from build123d import *

# Parameters (mm, degrees)
EXTRUDE_1_DEPTH                = 4
CUT_EXTRUDE_1_DEPTH            = 105.27847333
CUT_EXTRUDE_1_DEPTH_BACK       = 105.27847333
SKETCH_2_R                     = 2
SKETCH_2_W                     = 4
SKETCH_2_H                     = 16
CHAMFER_1_SIZE                 = 1
CUT_EXTRUDE_2_DEPTH            = 105.27847333
CUT_EXTRUDE_2_DEPTH_BACK       = 105.27847333
SKETCH_6_W                     = 20
SKETCH_6_H                     = 5
EXTRUDE_2_DEPTH                = 25
CHAMFER_2_SIZE                 = 1
EXTRUDE_START                  = -5
EXTRUDE_3_DEPTH                = 5
SKETCH_8_R                     = 6
EXTRUDE_4_DEPTH                = 5
CHAMFER_3_SIZE                 = 1
SKETCH_9_R                     = 4
EXTRUDE_5_DEPTH                = 5
CUT_EXTRUDE_START              = -10
SKETCH_10_R                    = 2
CUT_EXTRUDE_3_DEPTH            = 120.608393839
HOLE_WIZARD_1_4_0_15748031_1_D = 3.999999874
SKETCH_13_R                    = 1.5
CUT_EXTRUDE_4_DEPTH            = 109.434311913
SKETCH_14_R                    = 2
CUT_EXTRUDE_5_DEPTH            = 109.434311913
CUT_EXTRUDE_START_2            = 10
SKETCH_15_R                    = 4
CUT_EXTRUDE_6_DEPTH            = 10
CHAMFER_4_SIZE                 = 2
CHAMFER_5_SIZE                 = 1
SKETCH_16_W                    = 18
SKETCH_16_H                    = 4
CUT_EXTRUDE_7_DEPTH            = 109.434311913
SKETCH_17_R                    = 1.5
EXTRUDE_6_DEPTH                = 3


with BuildPart() as part:
    # 草图1 → 凸台-拉伸1 (new body)
    with BuildSketch(Plane(origin=(0, 0, 0), x_dir=(1, 0, 0), z_dir=(0, 1, 0))):
        Polygon((0, -34), (0, 34), (17, 47), (32, 47), (32, 34), (55, 34), (55, 47), (61, 47), (63, 45), (93, 45), (93, -45), (63, -45), (61, -47), (55, -47), (55, -34), (32, -34), (32, -47), (17, -47), align=None)
    extrude(amount=EXTRUDE_1_DEPTH)

    # 草图2 → 切除-拉伸1 (cut, two sides: drawn at the far end of the back side and taken through both)
    with BuildSketch(Plane(origin=(0, 4, 0), x_dir=(1, 0, 0), z_dir=(0, 1, 0)).offset(-CUT_EXTRUDE_1_DEPTH_BACK)):
        with Locations(Location((13, 10, 0), (0, 0, 270))):
            Circle(SKETCH_2_R)
        with Locations(Location((13, -10, 0), (0, 0, 90))):
            Circle(SKETCH_2_R)
        with Locations((6, 0)):
            Rectangle(SKETCH_2_W, SKETCH_2_H)
        Polygon((4, 12), (4, 26), (17, 36.408329997), (17, 33.205766921), (8, 26), (8, 12), align=None)
        Polygon((8, -26), (8, -12), (4, -12), (4, -26), (17, -36.408329997), (17, -33.205766921), align=None)
    extrude(amount=CUT_EXTRUDE_1_DEPTH + CUT_EXTRUDE_1_DEPTH_BACK, mode=Mode.SUBTRACT)

    # 倒角1
    chamfer_1_edges = [part.edges().sort_by_distance(p)[0] for p in [
        (8.5, 4, 40.5),
        (24.5, 4, 47),
        (8.5, 4, -40.5),
        (24.5, 4, -47),
        (0, 4, 0),
    ]]
    chamfer(chamfer_1_edges, length=CHAMFER_1_SIZE)

    # 草图3 → 切除-拉伸2 (cut, two sides: drawn at the far end of the back side and taken through both)
    with BuildSketch(Plane(origin=(0, 4, 0), x_dir=(1, 0, 0), z_dir=(0, 1, 0)).offset(-CUT_EXTRUDE_2_DEPTH_BACK)):
        Polygon((93, 22), (33, 22), (21, 10), (21, -10), (33, -22), (93, -22), align=None)
    extrude(amount=CUT_EXTRUDE_2_DEPTH + CUT_EXTRUDE_2_DEPTH_BACK, mode=Mode.SUBTRACT)

    # 草图6 → 凸台-拉伸2 (add)
    with BuildSketch(Plane(origin=(0, 4, 0), x_dir=(1, 0, 0), z_dir=(0, 1, 0))):
        with BuildLine():
            Line((21, 10), (21, 15))
            ThreePointArc((21, 15), (15, 21), (21, 27))
            Line((21, 27), (33, 27))
            Line((33, 27), (33, 22))
            Line((33, 22), (21, 10))
        make_face()
        with Locations((83, 24.5)):
            Rectangle(SKETCH_6_W, SKETCH_6_H)
    extrude_2 = extrude(amount=EXTRUDE_2_DEPTH)

    # 镜向1: 凸台-拉伸2 across plane
    add(extrude_2.mirror(Plane.XY))

    # 倒角2
    chamfer_2_edges = [part.edges().sort_by_distance(p)[0] for p in [
        (83, 4, -27),
        (73, 4, -24.5),
        (83, 4, 27),
        (73, 4, 24.5),
    ]]
    chamfer(chamfer_2_edges, length=CHAMFER_2_SIZE)

    # 草图7 → 凸台-拉伸3 (add)
    with BuildSketch(Plane(origin=(0, 29, 0), x_dir=(1, 0, 0), z_dir=(0, 1, 0)).offset(EXTRUDE_START)):
        with BuildLine():
            Line((93, 22), (93, 27))
            Line((93, 27), (73, 27))
            Line((73, 27), (73, 21))
            Line((73, 21), (53, 21))
            Line((53, 21), (53, 27))
            Line((53, 27), (33, 27))
            Line((33, 27), (21, 27))
            ThreePointArc((21, 27), (15, 21), (21, 15))
            Line((21, 15), (21, 10))
            Line((21, 10), (21, -10))
            Line((21, -10), (21, -15))
            ThreePointArc((21, -15), (15, -21), (21, -27))
            Line((21, -27), (33, -27))
            Line((33, -27), (53, -27))
            Line((53, -27), (53, -21))
            Line((53, -21), (73, -21))
            Line((73, -21), (73, -27))
            Line((73, -27), (93, -27))
            Line((93, -27), (93, -22))
            Line((93, -22), (93, 22))
        make_face()
    extrude(amount=EXTRUDE_3_DEPTH)

    # 草图8 → 凸台-拉伸4 (add)
    with BuildSketch(Plane(origin=(0, 29, 0), x_dir=(1, 0, 0), z_dir=(0, 1, 0))):
        with Locations(Location((21, 21, 0), (0, 0, 270))):
            Circle(SKETCH_8_R)
        with Locations(Location((21, -21, 0), (0, 0, 270))):
            Circle(SKETCH_8_R)
    extrude(amount=EXTRUDE_4_DEPTH)

    # 倒角3
    chamfer_3_edges = [part.edges().sort_by_distance(p)[0] for p in [
        (21, 34, -27),
        (21, 34, 15),
    ]]
    chamfer(chamfer_3_edges, length=CHAMFER_3_SIZE)

    # 草图9 → 凸台-拉伸5 (add)
    with BuildSketch(Plane(origin=(0, 29, 0), x_dir=(1, 0, 0), z_dir=(0, 1, 0))):
        with Locations(Location((83, 21, 0), (0, 0, 270))):
            Circle(SKETCH_9_R)
    extrude_5 = extrude(amount=EXTRUDE_5_DEPTH)

    # 草图10 → 切除-拉伸3 (cut)
    with BuildSketch(Plane(origin=(0, 34, 0), x_dir=(1, 0, 0), z_dir=(0, 1, 0)).offset(CUT_EXTRUDE_START)):
        with Locations(Location((83, 21, 0), (0, 0, 270))):
            Circle(SKETCH_10_R)
    cut_extrude_3 = extrude(amount=CUT_EXTRUDE_3_DEPTH, mode=Mode.SUBTRACT)

    # 镜向2: 凸台-拉伸5, 切除-拉伸3 across plane
    add(extrude_5.mirror(Plane.XY))
    add(cut_extrude_3.mirror(Plane.XY), mode=Mode.SUBTRACT)

    # 1/4 (0.15748031) 直径孔1 (through all)
    with Locations(Plane(origin=(21, 34, -21), x_dir=(0, 0, 1), z_dir=(0, 1, 0))):
        with Locations((0, 0)):
            hole_wizard_1_4_0_15748031_1 = Hole(HOLE_WIZARD_1_4_0_15748031_1_D / 2)

    # 镜向3: 1/4 (0.15748031) 直径孔1 across plane
    add(hole_wizard_1_4_0_15748031_1.mirror(Plane.XY), mode=Mode.SUBTRACT)

    # 草图13 → 切除-拉伸4 (cut, symmetric)
    with BuildSketch(Plane(origin=(0, 4, 0), x_dir=(1, 0, 0), z_dir=(0, 1, 0))):
        with Locations(Location((29, 40, 0), (0, 0, 270))):
            Circle(SKETCH_13_R)
        with Locations(Location((58, 40, 0), (0, 0, 270))):
            Circle(SKETCH_13_R)
    cut_extrude_4 = extrude(amount=CUT_EXTRUDE_4_DEPTH, both=True, mode=Mode.SUBTRACT)

    # 镜向4: 切除-拉伸4 across plane
    add(cut_extrude_4.mirror(Plane.XY), mode=Mode.SUBTRACT)

    # 草图14 → 切除-拉伸5 (cut, symmetric)
    with BuildSketch(Plane(origin=(0, 4, 0), x_dir=(1, 0, 0), z_dir=(0, 1, 0))):
        with Locations(Location((63, 27, 0), (0, 0, 270))):
            Circle(SKETCH_14_R)
    cut_extrude_5 = extrude(amount=CUT_EXTRUDE_5_DEPTH, both=True, mode=Mode.SUBTRACT)

    # 镜向5: 切除-拉伸5 across plane
    add(cut_extrude_5.mirror(Plane.XY), mode=Mode.SUBTRACT)

    # 草图15 → 切除-拉伸6 (cut)
    with BuildSketch(Plane.XZ.offset(-24).offset(CUT_EXTRUDE_START_2)):
        with Locations(Location((83, 21, 0), (0, 0, 270))):
            Circle(SKETCH_15_R)
        with Locations(Location((83, -21, 0), (0, 0, 90))):
            Circle(SKETCH_15_R)
    extrude(amount=-CUT_EXTRUDE_6_DEPTH, mode=Mode.SUBTRACT)

    # 倒角4
    chamfer_4_edges = [part.edges().sort_by_distance(p)[0] for p in [
        (83, 24, -23),
        (83, 24, 23),
    ]]
    chamfer(chamfer_4_edges, length=CHAMFER_4_SIZE - 0.0001)  # a hair under: the kernel refuses the full size

    # 倒角5
    chamfer_5_edges = [part.edges().sort_by_distance(p)[0] for p in [
        (83, 34, -25),
        (83, 34, 25),
    ]]
    chamfer(chamfer_5_edges, length=CHAMFER_5_SIZE)

    # 草图16 → 切除-拉伸7 (cut, through all)
    with BuildSketch(Plane(origin=(0, 4, 0), x_dir=(1, 0, 0), z_dir=(0, 1, 0))):
        with Locations((84, 39)):
            Rectangle(SKETCH_16_W, SKETCH_16_H)
    cut_extrude_7 = extrude(amount=-CUT_EXTRUDE_7_DEPTH, mode=Mode.SUBTRACT)

    # 镜向6: 切除-拉伸7 across plane
    add(cut_extrude_7.mirror(Plane.XY), mode=Mode.SUBTRACT)

    # 草图17 → 凸台-拉伸6 (add)
    with BuildSketch(Plane(origin=(93, 0, 0), x_dir=(0, 0, -1), z_dir=(1, 0, 0))):
        with Locations(Location((24.5, 4, 0), (0, 0, 180))):
            Circle(SKETCH_17_R)
    extrude_6 = extrude(amount=EXTRUDE_6_DEPTH)

    # 镜向7: 凸台-拉伸6 across plane
    add(extrude_6.mirror(Plane.XY))


solid = part.part
Verification items for the finished model (mm, model axes). A direction names the side the tool comes from. Give positions to 0.01 mm unless a question says otherwise; leave off trailing zeros. Write each loop counter-clockwise with the first axis right and the second up, starting at its lowest first coordinate (ties: lowest second). Pieces come first, ordered by that corner, then holes. Notation, with made-up numbers: M -23,-8 L 17,-8 A10 cw 17,-1 Z; hole C 67.5,32 d9. An arc over 180 degrees is marked long. Put each result on its own line as item: value. Start each with the question number.
1. Draft check along X on faces 6 (the face through (4, 2, 19)), 7 (the face through (24, 1, -47)), 8 (the face through (0, 1, 0)). Enter one of: +X half, -X half, draft (parallel to the pull), parting line (faces both ways), or undercut.
2. Set-up check for faces 1 (the face through (84, 2, 37)), 2 (the face through (32, 2, 40)), 3 (the face through (56, 29, 0)), 4 (the face through (10.41, 1.97, 31.13)), 5 (the face through (55, 2, -40)): record each of +Z, -Z, +X, -X, +Y, -Y from which the full face is reachable in a straight line by a thin tool's end or side.
3. Section check D-D (x = 13). Record the cut outline in (y, z), and give its area (3 significant figures).
4. Section check C-C (z = 5). Record the cut outline in (x, y), and give its area (4 significant figures).
5. Section check B-B (x = 37). Record the cut outline in (y, z).
6. Scan lines: line 1 along X through (y, z) = (1.35, 10); line 2 along X through (y, z) = (17.5, -21); line 3 along Z through (x, y) = (77.5, 19). Record each from-to range of solid material in increasing order. Write a range as [from, to].
7. Section check A-A (y = 19.5). Record the cut outline in (x, z), and give its area (3 significant figures).
8. Go/stop test with flat-tipped pins: pin 1 Ø2 at (x, z) = (29, -5.5) entering from -Y; pin 2 Ø3 at (y, z) = (5, -16) entering from -X; pin 3 Ø4 at (x, y) = (49.5, 5) entering from +Z. Record where each tip stops, or that it passes through.
Answer list:
1. face 6: undercut
1. face 7: draft
1. face 8: -X half
2. face 1: +X, +Y, -Y
2. face 2: +Z, +Y, -Y
2. face 3: +Y
2. face 4: +Y, -Y
2. face 5: -Z, +Y, -Y
3. outline: M 0,-43.94 L 3,-43.94 L 4,-42.68 L 4,-33.21 L 0,-33.21 Z; M 0,-30 L 4,-30 L 4,-12 L 0,-12 Z; M 0,-8 L 4,-8 L 4,8 L 0,8 Z; M 0,12 L 4,12 L 4,30 L 0,30 Z; M 0,33.21 L 4,33.21 L 4,42.68 L 3,43.94 L 0,43.94 Z
3. area: 293 mm2
4. outline: M 0,0 L 4,0 L 4,4 L 1,4 L 0,3 Z; M 8,0 L 21,0 L 21,4 L 8,4 Z; M 21,24 L 93,24 L 93,29 L 21,29 Z
4. area: 427.5 mm2
5. outline: M 0,-34 L 4,-34 L 4,-22 L 0,-22 Z; M 0,22 L 4,22 L 4,34 L 0,34 Z; M 24,-27 L 29,-27 L 29,27 L 24,27 Z
6. line 1: [0, 11], [15, 21]
6. line 2: [15, 19], [23, 32]
6. line 3: [-27, -22], [22, 27]
7. outline: M 21,-27 L 33,-27 L 33,-22 L 21,-10 L 21,-15 A6 ccw Z; M 21,10 L 33,22 L 33,27 L 21,27 A6 ccw 21,15 Z; M 73,-27 L 93,-27 L 93,-22 L 86.87,-22 A4 cw 79.13,-22 L 73,-22 Z; M 73,22 L 79.13,22 A4 cw 86.87,22 L 93,22 L 93,27 L 73,27 Z; hole C 21,-21 d4; hole C 21,21 d4
7. area: 518 mm2
8. pin 1: y = 24
8. pin 2: x = 0.5
8. pin 3: z = 34
